Could you check a few things on this model? Use its own coordinates, in mm. A direction names the side the tool comes from. Round coordinates to 2 decimals unless told otherwise and drop trailing zeros. Loops run counter-clockwise (first coordinate to the right, second up) from the corner with the lowest first, then second, coordinate; pieces in that order, holes last. Notation, with made-up numbers: M 82,3 L 124,3 A16 ccw 124,16 Z; hole C 35.25,-21 d9. An arc over 180 degrees is marked long. Answer in a Markdown table with one row per item.
```python
from build123d import *

# Parameters (mm, degrees)
EXTRUDE_1_DEPTH = 10
SKETCH_3_R      = 5
EXTRUDE_2_DEPTH = 24


with BuildPart() as part:
    # 草图1 → 凸台-拉伸1 (new body)
    with BuildSketch(Plane(origin=(0, 0, 0), x_dir=(1, 0, 0), z_dir=(0, 1, 0))):
        with BuildLine():
            Line((0, 15), (36, 15))
            Line((36, 15), (36, 41))
            Line((36, 41), (60, 41))
            Line((60, 41), (60, -5))
            Line((60, -5), (40, -15))
            Line((40, -15), (0, -15))
            ThreePointArc((0, -15), (-15, 0), (0, 15))
        make_face()
        with BuildLine():
            Line((0, 6), (22, 6))
            ThreePointArc((22, 6), (28, 0), (22, -6))
            Line((22, -6), (0, -6))
            ThreePointArc((0, -6), (-6, 0), (0, 6))
        make_face(mode=Mode.SUBTRACT)
    extrude(amount=EXTRUDE_1_DEPTH)

    # 草图3 → 凸台-拉伸2 (add)
    with BuildSketch(Plane(origin=(60, 0, 0), x_dir=(0, 0, -1), z_dir=(1, 0, 0))):
        with BuildLine():
            Line((41, 10), (21, 10))
            Line((21, 10), (21, 35))
            ThreePointArc((21, 35), (31, 45), (41, 35))
            Line((41, 35), (41, 10))
        make_face()
        with Locations((31, 35)):
            Circle(SKETCH_3_R, mode=Mode.SUBTRACT)
    extrude(amount=-EXTRUDE_2_DEPTH)


solid = part.part
```
1) If we mould it in two halves opening along Y, with no side actions, what happens to faces 1 (the face through (48, 35, -26)), 2 (the face through (31, 10, -3)), 3 (the face through (48, 22, -21))? For each: released by +Y, released by -Y, zero draft, split by the parting line, or undercut.
Computed:
| item | result |
|---|---|
| face 1 | undercut |
| face 2 | released by +Y |
| face 3 | zero draft |
2) I want a section at B-B, the plane x = 14.5. Please give me the cut outline in (y, z).
Computed:
| item | result |
|---|---|
| outline | M 0,-15 L 10,-15 L 10,-6 L 0,-6 Z; M 0,6 L 10,6 L 10,15 L 0,15 Z |
3) I want a section at D-D, the plane y = 12. Please give me the cut outline in (x, z), plus the area to 3 significant figures.
Computed:
| item | result |
|---|---|
| outline | M 36,-41 L 60,-41 L 60,-21 L 36,-21 Z |
| area | 480 mm² |
4) I want a section at A-A, the plane z = -31. Please give me the cut outline in (x, y).
Computed:
| item | result |
|---|---|
| outline | M 36,0 L 60,0 L 60,30 L 36,30 Z; M 36,40 L 60,40 L 60,45 L 36,45 Z |
5) Which directions (+Z, -Z, +X, -X, +Y, -Y) give clear straight access to the entire face, cutting with the end or side of a thin tool? Please do faces 4 (the face through (50, 5, 10)), 5 (the face through (11, 5, -6)), 6 (the face through (36, 18, -31)).
Computed:
| item | result |
|---|---|
| face 4 | +Z, +X, +Y, -Y |
| face 5 | +Y, -Y |
| face 6 | -Z, -X, +Y, -Y |
6) I want a section at C-C, the plane y = 5. Please give me the cut outline in (x, z), plus the area to 3 significant figures.
Computed:
| item | result |
|---|---|
| outline | M 0,-15 L 36,-15 L 36,-41 L 60,-41 L 60,5 L 40,15 L 0,15 A15 ccw Z; hole M 0,-6 L 22,-6 A6 ccw 22,6 L 0,6 A6 ccw Z |
| area | 2,300 mm² |
7) I need wall thicknesses on line 1 (Z direction, x = 18, y = 3); line 2 (Y direction, x = 55, z = -31); line 3 (Y direction, x = 53.5, z = -8.5). Which ranges of each line are inside material? Lowest first, please.
Computed:
| item | result |
|---|---|
| line 1 | z = -15 to -6, 6 to 15 |
| line 2 | y = 0 to 30, 40 to 45 |
| line 3 | y = 0 to 10 |
8) Will these pins go through, and if not, where does the flat tip stop? P1, Ø11.5, axis at y = 35, z = -31, coming from the -X side; P2, Ø1.5, axis at x = 28, z = -3.5, coming from the +Y side; P3, Ø3, axis at x = 21, y = 5.5, coming from the -Z side.
Computed:
| item | result |
|---|---|
| P1 | stops at x = 36 |
| P2 | stops at y = 10 |
| P3 | stops at z = -15 |
